```python
from build123d import *

# Parameters (mm, degrees)
F0_W     = 80
F0_H     = 80
F0_R     = 21.5
F1_DEPTH = 20
F3_DEPTH = 16


with BuildPart() as f1:
    # F0 (on Top) → F1 (new body)
    with BuildSketch(Plane.XY):
        with Locations((40, -40)):
            Rectangle(F0_W, F0_H)
        with Locations((40, -40)):
            Circle(F0_R, mode=Mode.SUBTRACT)
    extrude(amount=F1_DEPTH)

    # F2 (on face) → F3 (cut)
    with BuildSketch(Plane(origin=(0, 0, 0), x_dir=(-1, 0, 0), z_dir=(0, 1, 0))):
        with BuildLine():
            ThreePointArc((-64, 10), (-68, 14), (-72, 10))
            Line((-72, 10), (-64, 10))
        make_face()
        with BuildLine():
            Line((-64, 10), (-72, 10))
            ThreePointArc((-72, 10), (-68, 6), (-64, 10))
        make_face()
        with BuildLine():
            ThreePointArc((-16, 10), (-12, 6), (-8, 10))
            Line((-8, 10), (-16, 10))
        make_face()
        with BuildLine():
            Line((-16, 10), (-8, 10))
            ThreePointArc((-8, 10), (-12, 14), (-16, 10))
        make_face()
        with BuildLine():
            Line((-44, 10), (-36, 10))
            ThreePointArc((-36, 10), (-40, 14), (-44, 10))
        make_face()
        with BuildLine():
            ThreePointArc((-44, 10), (-40, 6), (-36, 10))
            Line((-36, 10), (-44, 10))
        make_face()
    extrude(amount=-F3_DEPTH, mode=Mode.SUBTRACT)


solid = f1.part
```
Design review of the part built by this model. Coordinates are the model's own, in mm. A direction names the side the tool comes from. Coordinates: 2 decimals unless noted, no trailing zeros. Loops run counter-clockwise (first coordinate to the right, second up) from the corner with the lowest first, then second, coordinate; pieces in that order, holes last. Notation, with made-up numbers: M 41.5,-21 L 55.5,-21 A32 cw 55.5,5 Z; hole C 55.5,31 d9. An arc over 180 degrees is marked long. One line per question, with ' | ' between items.
(1) We need section A-A (z = 10). Give the boundary of the cut face in (x, y), and give its area (3 significant figures).
Filled in:
outline: M 0,-80 L 80,-80 L 80,0 L 72,0 L 72,-16 L 64,-16 L 64,0 L 44,0 L 44,-16 L 36,-16 L 36,0 L 16,0 L 16,-16 L 8,-16 L 8,0 L 0,0 Z; hole C 40,-40 d43 | area: 4,560 mm^2
(2) Draft analysis for pull direction Y (two halves, no side actions). For faces 3 (the face through (35.34, -60.99, 9.86)), 4 (the face through (39, 0, 5)), 5 (the face through (80, -41, 10)), state which applies: released by +Y, released by -Y, zero draft, split by the parting line, or undercut.
Filled in:
face 3: undercut | face 4: released by +Y | face 5: zero draft
(3) We need section C-C (y = -53.5). Give the boundary of the cut face in (x, z).
Filled in:
outline: M 0,0 L 23.27,0 L 23.27,20 L 0,20 Z; M 56.73,0 L 80,0 L 80,20 L 56.73,20 Z
(4) We need section D-D (y = -9). Give the boundary of the cut face in (x, z).
Filled in:
outline: M 0,0 L 80,0 L 80,20 L 0,20 Z; hole C 12,10 d8; hole C 40,10 d8; hole C 68,10 d8
(5) For pin 1 Ø6.5 at (x, z) = (11.5, 10) entering from +Y, flat-tipped, find the tip position at first contact; note if it passes through.
Filled in:
pin 1: stops at y = -16
(6) We need section B-B (x = 40). Give the boundary of the cut face in (y, z), and give its area (3 significant figures).
Filled in:
outline: M -80,0 L -61.5,0 L -61.5,20 L -80,20 Z; M -18.5,0 L 0,0 L 0,6 L -16,6 L -16,14 L 0,14 L 0,20 L -18.5,20 Z | area: 612 mm^2
(7) Machinability: for faces 1 (the face through (36.8, -7.9, 12.4)), 2 (the face through (0, -41, 10)), which of the approach directions +Z, -Z, +X, -X, +Y, -Y give a long, thin tool a straight path to every point of the face, cutting with its end or side? Answer none if there is none.
Filled in:
face 1: +Y | face 2: +Z, -Z, -X, +Y, -Y
(8) Wall thickness on probe 1 along Y at (x, z) = (40, 9.75); probe 2 along Z at (x, y) = (12, -4.5); probe 3 along X at (y, z) = (-38, 8): over which ranges is each line inside the solid? List them lowest first.
Filled in:
probe 1: y = -80 to -61.5, -18.5 to -16 | probe 2: z = 0 to 6, 14 to 20 | probe 3: x = 0 to 18.59, 61.41 to 80
